Could you check a few things on this drawing? It's one solid part, dimensions in mm from its lowest x, y, z. Coordinates: 2 decimals unless noted, no trailing zeros. Write each loop counter-clockwise with the first axis right and the second up, starting at its lowest first coordinate (ties: lowest second). Pieces come first, ordered by that corner, then holes. Notation, with made-up numbers: (-10.75, 2.25) - (7.25, 2.25) arc R17 cw to (7.25, 6.25) - close; hole circle Ø7 at (9.25, 82). An arc over 180 degrees is marked (long way). Answer as a JSON object with one key per item and string values. Group by question number.
1) If we section it at D-D (x = 18.5): Write out the boundary of the cut face in (y, z), plus the area to 3 significant figures.
2) If we section it at A-A (z = 55): Write out the boundary of the cut face in (x, y), plus the area to 3 significant figures.
3) We'd pull the mould along Z, two halves only. Please class the marked faces 1, 2, 3 and 4: released by +Z, released by -Z, zero draft, split by the parting line, or undercut.
4) Will these pins go through, and if not, where does the flat tip stop? pin 1 Ø8 at (x, y) = (70, 27) entering from -Z (3 decimals); pin 2 Ø5 at (x, y) = (60, 8.5) entering from -Z; pin 3 Ø8 at (x, y) = (47.5, 9) entering from +Z; pin 4 Ø4 at (x, z) = (15, 31.5) entering from -Y.
5) If we section it at C-C (x = 55): Write out the boundary of the cut face in (y, z).
6) Please list where these lines run through material, in increasing order: line 1 along X through (y, z) = (19.5, 55); line 2 along X through (y, z) = (14.75, 71.5); line 3 along Z through (x, y) = (73.5, 4).
7) If we section it at B-B (y = 4.5): Write out the boundary of the cut face in (x, z), plus the area to 3 significant figures.
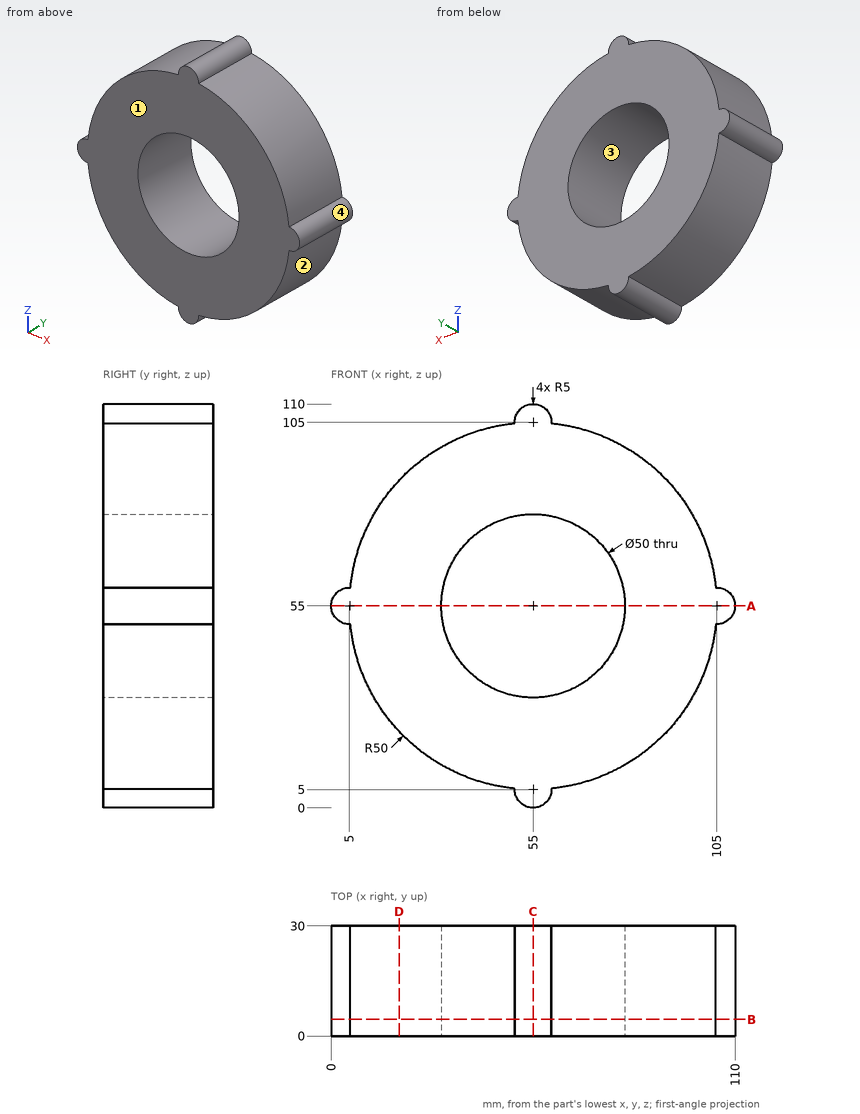
Here are the results:
{
 "1": {"outline": "(0, 20.83) - (30, 20.83) - (30, 89.17) - (0, 89.17) - close", "area": "2,050 mm²"},
 "2": {"outline": "(0, 0) - (30, 0) - (30, 30) - (0, 30) - close; (80, 0) - (110, 0) - (110, 30) - (80, 30) - close", "area": "1,800 mm²"},
 "3": {"face 1": "zero draft", "face 2": "released by -Z", "face 3": "undercut", "face 4": "split by the parting line"},
 "4": {"pin 1": "stops at z = 6.225", "pin 2": "stops at z = 0.67", "pin 3": "stops at z = 108.57", "pin 4": "stops at y = 0"},
 "5": {"outline": "(0, 0) - (30, 0) - (30, 30) - (0, 30) - close; (0, 80) - (30, 80) - (30, 110) - (0, 110) - close"},
 "6": {"line 1": "x = 0 to 30, 80 to 110", "line 2": "x = 7.8 to 36.22, 73.78 to 102.2", "line 3": "z = 8.55 to 38.18, 71.82 to 101.45"},
 "7": {"outline": "(5.25, 50.01) arc R50 ccw to (50.01, 5.25) arc R5 ccw (long way) to (59.99, 5.25) arc R50 ccw to (104.75, 50.01) arc R5 ccw (long way) to (104.75, 59.99) arc R50 ccw to (59.99, 104.75) arc R5 ccw (long way) to (50.01, 104.75) arc R50 ccw to (5.25, 59.99) arc R5 ccw (long way) to start; hole circle Ø50 at (55, 55)", "area": "6,050 mm²"}
}
